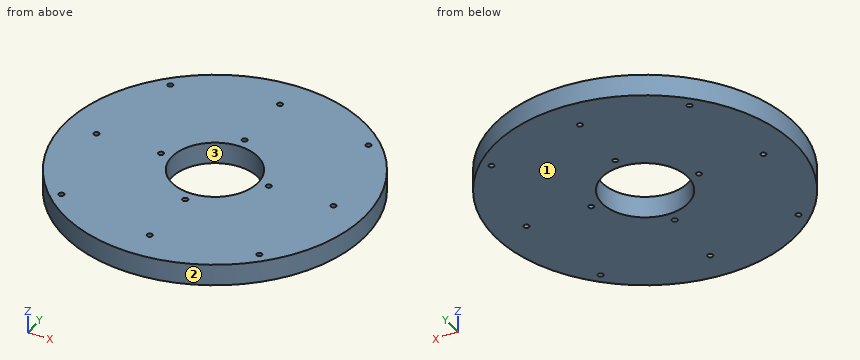
```python
from build123d import *

# Parameters (mm, degrees)
F0_R     = 140
F1_DEPTH = 20
F3_DEPTH = 20.001
F5_DEPTH = 25
F6_R     = 40
F7_DEPTH = 25
F9_DEPTH = 25


with BuildPart() as f1:
    # F0 (on Top) → F1 (new body)
    with BuildSketch(Plane.XY):
        Circle(F0_R)
    extrude(amount=F1_DEPTH)

    # F2 (on face) → F3 (cut, through all)
    with BuildSketch(Plane.XY.offset(20)):
        with BuildLine():
            ThreePointArc((-2.4998385795, 109.9715909091), (0, 110), (2.4998385795, 109.9715909091))
            ThreePointArc((2.4998385795, 109.9715909091), (2.4999596445, 109.9857952252), (2.5, 110))
            ThreePointArc((2.5, 110), (-0.0142047748, 112.4999596445), (-2.4998385795, 109.9715909091))
        make_face()
        with BuildLine():
            ThreePointArc((-2.4998385795, 109.9715909091), (0, 107.5), (2.4998385795, 109.9715909091))
            ThreePointArc((2.4998385795, 109.9715909091), (0, 110), (-2.4998385795, 109.9715909091))
        make_face()
        with BuildLine():
            ThreePointArc((109.9715909091, 2.4998385795), (109.992897498, 1.25), (110, 0))
            ThreePointArc((110, 0), (109.992897498, -1.25), (109.9715909091, -2.4998385795))
            ThreePointArc((109.9715909091, -2.4998385795), (111.7576941248, -1.7777827099), (112.5, 0))
            ThreePointArc((112.5, 0), (111.7576941248, 1.7777827099), (109.9715909091, 2.4998385795))
        make_face()
        with BuildLine():
            ThreePointArc((109.9715909091, -2.4998385795), (109.992897498, -1.25), (110, 0))
            ThreePointArc((110, 0), (109.992897498, 1.25), (109.9715909091, 2.4998385795))
            ThreePointArc((109.9715909091, 2.4998385795), (107.5, 0), (109.9715909091, -2.4998385795))
        make_face()
        with BuildLine():
            ThreePointArc((2.5, -110), (2.4999596445, -109.9857952252), (2.4998385795, -109.9715909091))
            ThreePointArc((2.4998385795, -109.9715909091), (0, -110), (-2.4998385795, -109.9715909091))
            ThreePointArc((-2.4998385795, -109.9715909091), (-0.0142047748, -112.4999596445), (2.5, -110))
        make_face()
        with BuildLine():
            ThreePointArc((-2.4998385795, -109.9715909091), (0, -110), (2.4998385795, -109.9715909091))
            ThreePointArc((2.4998385795, -109.9715909091), (0, -107.5), (-2.4998385795, -109.9715909091))
        make_face()
        with BuildLine():
            ThreePointArc((-107.5, 0), (-108.2222172901, 1.7576941248), (-109.9715909091, 2.4998385795))
            ThreePointArc((-109.9715909091, 2.4998385795), (-110, 0), (-109.9715909091, -2.4998385795))
            ThreePointArc((-109.9715909091, -2.4998385795), (-108.2222172901, -1.7576941248), (-107.5, 0))
        make_face()
        with BuildLine():
            ThreePointArc((-109.9715909091, -2.4998385795), (-110, 0), (-109.9715909091, 2.4998385795))
            ThreePointArc((-109.9715909091, 2.4998385795), (-112.5, 0), (-109.9715909091, -2.4998385795))
        make_face()
    extrude(amount=-F3_DEPTH, mode=Mode.SUBTRACT)

    # F4 (on face) → F5 (cut)
    with BuildSketch(Plane.XY.offset(20)):
        with BuildLine():
            ThreePointArc((-89.4238815543, 91.9238815543), (-89.6096098032, 92.8694746286), (-90.139198564, 93.6745690262))
            ThreePointArc((-90.139198564, 93.6745690262), (-91.0357485398, 92.8035154927), (-91.9238815543, 91.9238815543))
            Line((-91.9238815543, 91.9238815543), (-90.1561146013, 90.1561146013))
            ThreePointArc((-90.1561146013, 90.1561146013), (-89.614182723, 90.9671729733), (-89.4238815543, 91.9238815543))
        make_face()
        with BuildLine():
            ThreePointArc((-93.6745690262, 90.139198564), (-91.9118621846, 89.4239104475), (-90.1561146013, 90.1561146013))
            Line((-90.1561146013, 90.1561146013), (-91.9238815543, 91.9238815543))
            ThreePointArc((-91.9238815543, 91.9238815543), (-92.8035154927, 91.0357485398), (-93.6745690262, 90.139198564))
        make_face()
        with BuildLine():
            ThreePointArc((-91.9238815543, 91.9238815543), (-91.0357485398, 92.8035154927), (-90.139198564, 93.6745690262))
            ThreePointArc((-90.139198564, 93.6745690262), (-93.6916485072, 93.6916485072), (-93.6745690262, 90.139198564))
            ThreePointArc((-93.6745690262, 90.139198564), (-92.8035154927, 91.0357485398), (-91.9238815543, 91.9238815543))
        make_face()
        with BuildLine():
            ThreePointArc((91.9238815543, 91.9238815543), (92.8035154927, 91.0357485398), (93.6745690262, 90.139198564))
            ThreePointArc((93.6745690262, 90.139198564), (94.228954078, 90.9560795807), (94.4238815543, 91.9238815543))
            ThreePointArc((94.4238815543, 91.9238815543), (92.8694746286, 94.2381533053), (90.139198564, 93.6745690262))
            ThreePointArc((90.139198564, 93.6745690262), (91.0357485398, 92.8035154927), (91.9238815543, 91.9238815543))
        make_face()
        with BuildLine():
            ThreePointArc((90.1561146013, 90.1561146013), (91.9118621846, 89.4239104475), (93.6745690262, 90.139198564))
            ThreePointArc((93.6745690262, 90.139198564), (92.8035154927, 91.0357485398), (91.9238815543, 91.9238815543))
            Line((91.9238815543, 91.9238815543), (90.1561146013, 90.1561146013))
        make_face()
        with BuildLine():
            Line((90.1561146013, 90.1561146013), (91.9238815543, 91.9238815543))
            ThreePointArc((91.9238815543, 91.9238815543), (91.0357485398, 92.8035154927), (90.139198564, 93.6745690262))
            ThreePointArc((90.139198564, 93.6745690262), (89.4239104475, 91.9118621846), (90.1561146013, 90.1561146013))
        make_face()
        with BuildLine():
            ThreePointArc((94.4238815543, -91.9238815543), (94.228954078, -90.9560795807), (93.6745690262, -90.139198564))
            ThreePointArc((93.6745690262, -90.139198564), (92.8035154927, -91.0357485398), (91.9238815543, -91.9238815543))
            ThreePointArc((91.9238815543, -91.9238815543), (91.0357485398, -92.8035154927), (90.139198564, -93.6745690262))
            ThreePointArc((90.139198564, -93.6745690262), (92.8694746286, -94.2381533053), (94.4238815543, -91.9238815543))
        make_face()
        with BuildLine():
            ThreePointArc((91.9238815543, -91.9238815543), (92.8035154927, -91.0357485398), (93.6745690262, -90.139198564))
            ThreePointArc((93.6745690262, -90.139198564), (91.9118621846, -89.4239104475), (90.1561146013, -90.1561146013))
            Line((90.1561146013, -90.1561146013), (91.9238815543, -91.9238815543))
        make_face()
        with BuildLine():
            ThreePointArc((90.139198564, -93.6745690262), (91.0357485398, -92.8035154927), (91.9238815543, -91.9238815543))
            Line((91.9238815543, -91.9238815543), (90.1561146013, -90.1561146013))
            ThreePointArc((90.1561146013, -90.1561146013), (89.4239104475, -91.9118621846), (90.139198564, -93.6745690262))
        make_face()
        with BuildLine():
            ThreePointArc((-89.4238815543, -91.9238815543), (-89.614182723, -90.9671729733), (-90.1561146013, -90.1561146013))
            Line((-90.1561146013, -90.1561146013), (-91.9238815543, -91.9238815543))
            ThreePointArc((-91.9238815543, -91.9238815543), (-91.0357485398, -92.8035154927), (-90.139198564, -93.6745690262))
            ThreePointArc((-90.139198564, -93.6745690262), (-89.6096098032, -92.8694746286), (-89.4238815543, -91.9238815543))
        make_face()
        with BuildLine():
            ThreePointArc((-93.6745690262, -90.139198564), (-93.6916485072, -93.6916485072), (-90.139198564, -93.6745690262))
            ThreePointArc((-90.139198564, -93.6745690262), (-91.0357485398, -92.8035154927), (-91.9238815543, -91.9238815543))
            ThreePointArc((-91.9238815543, -91.9238815543), (-92.8035154927, -91.0357485398), (-93.6745690262, -90.139198564))
        make_face()
        with BuildLine():
            Line((-91.9238815543, -91.9238815543), (-90.1561146013, -90.1561146013))
            ThreePointArc((-90.1561146013, -90.1561146013), (-91.9118621846, -89.4239104475), (-93.6745690262, -90.139198564))
            ThreePointArc((-93.6745690262, -90.139198564), (-92.8035154927, -91.0357485398), (-91.9238815543, -91.9238815543))
        make_face()
    extrude(amount=-F5_DEPTH, mode=Mode.SUBTRACT)

    # F6 (on face) → F7 (cut)
    with BuildSketch(Plane.XY.offset(20)):
        Circle(F6_R)
    extrude(amount=-F7_DEPTH, mode=Mode.SUBTRACT)

    # F8 (on face) → F9 (cut)
    with BuildSketch(Plane.XY.offset(20)):
        with BuildLine():
            ThreePointArc((-2.4992186279, 49.9375), (0, 50), (2.4992186279, 49.9375))
            ThreePointArc((2.4992186279, 49.9375), (2.4998046493, 49.9687475579), (2.5, 50))
            ThreePointArc((2.5, 50), (-0.0312524421, 52.4998046493), (-2.4992186279, 49.9375))
        make_face()
        with BuildLine():
            ThreePointArc((-2.4992186279, 49.9375), (0, 47.5), (2.4992186279, 49.9375))
            ThreePointArc((2.4992186279, 49.9375), (0, 50), (-2.4992186279, 49.9375))
        make_face()
        with BuildLine():
            ThreePointArc((-47.5, 0), (-48.2102723671, 1.7455300055), (-49.9375, 2.4992186279))
            ThreePointArc((-49.9375, 2.4992186279), (-50, 0), (-49.9375, -2.4992186279))
            ThreePointArc((-49.9375, -2.4992186279), (-48.2102723671, -1.7455300055), (-47.5, 0))
        make_face()
        with BuildLine():
            ThreePointArc((-49.9375, -2.4992186279), (-50, 0), (-49.9375, 2.4992186279))
            ThreePointArc((-49.9375, 2.4992186279), (-52.5, 0), (-49.9375, -2.4992186279))
        make_face()
        with BuildLine():
            ThreePointArc((2.5, -50), (2.4998046493, -49.9687475579), (2.4992186279, -49.9375))
            ThreePointArc((2.4992186279, -49.9375), (0, -50), (-2.4992186279, -49.9375))
            ThreePointArc((-2.4992186279, -49.9375), (-0.0312524421, -52.4998046493), (2.5, -50))
        make_face()
        with BuildLine():
            ThreePointArc((-2.4992186279, -49.9375), (0, -50), (2.4992186279, -49.9375))
            ThreePointArc((2.4992186279, -49.9375), (0, -47.5), (-2.4992186279, -49.9375))
        make_face()
        with BuildLine():
            ThreePointArc((49.9375, 2.4992186279), (49.9843725578, 1.25), (50, 0))
            ThreePointArc((50, 0), (49.9843725578, -1.25), (49.9375, -2.4992186279))
            ThreePointArc((49.9375, -2.4992186279), (51.7455300055, -1.7897276329), (52.5, 0))
            ThreePointArc((52.5, 0), (51.7455300055, 1.7897276329), (49.9375, 2.4992186279))
        make_face()
        with BuildLine():
            ThreePointArc((49.9375, -2.4992186279), (49.9843725578, -1.25), (50, 0))
            ThreePointArc((50, 0), (49.9843725578, 1.25), (49.9375, 2.4992186279))
            ThreePointArc((49.9375, 2.4992186279), (47.5, 0), (49.9375, -2.4992186279))
        make_face()
    extrude(amount=-F9_DEPTH, mode=Mode.SUBTRACT)


solid = f1.part
```
Check sheet for the modelled part. Datum: model origin and axes. Units: mm. Face numbers are marked on the shaded views. Coordinates: 2 decimals unless noted, no trailing zeros. Order: outer loops, then holes, each group sorted by start corner. A loop starts at its lowest first (then second) coordinate and runs counter-clockwise, first axis right, second up. Notation, with made-up numbers: M 22.25,49 L 30.25,49 A32 ccw 30.25,78 Z; hole C 72,74 d7. An arc over 180 degrees is marked long. Write each question's results on one line, items separated by ' | '. Start each with the question number.
1. Cross-section at D-D on x = -69. Record the cut outline in (y, z), and give its area (3 significant figures).
2. Cross-section at C-C on y = -70. Record the cut outline in (x, z), and give its area (3 significant figures).
3. Go/stop test with flat-tipped pins: P1, Ø4, axis at x = -102.5, z = 6, coming from the +Y side; P2, Ø6, axis at x = -32, z = 11, coming from the +Y side; P3, Ø5, axis at x = 4.5, z = 17.5, coming from the -Y side. Record where each tip stops, or that it passes through.
4. Cross-section at A-A on x = -16.5. Record the cut outline in (y, z).
5. Cross-section at B-B on y = 7. Record the cut outline in (x, z).
6. Mould release check, pull along X, two halves, no side actions. Record for the marked faces 1, 2 and 3: +X half, -X half, draft (parallel to the pull), parting line (faces both ways), or undercut.
7. Material ranges on probe 1 along X at (y, z) = (50.5, 10.75); probe 2 along Y at (x, z) = (-10.5, 3.75); probe 3 along X at (y, z) = (6.5, 17.75), recorded low to high.
Checks:
1) outline: M -121.82,0 L 121.82,0 L 121.82,20 L -121.82,20 Z | area: 4,870 mm²
2) outline: M -121.24,0 L 121.24,0 L 121.24,20 L -121.24,20 Z | area: 4,850 mm²
3) P1: stops at y = 97.47 | P2: stops at y = 136.96 | P3: stops at y = -139.99
4) outline: M -139.02,0 L -36.44,0 L -36.44,20 L -139.02,20 Z; M 36.44,0 L 139.02,0 L 139.02,20 L 36.44,20 Z
5) outline: M -139.82,0 L -39.38,0 L -39.38,20 L -139.82,20 Z; M 39.38,0 L 139.82,0 L 139.82,20 L 39.38,20 Z
6) face 1: draft | face 2: parting line | face 3: undercut
7) probe 1: x = -130.57 to -2.45, 2.45 to 130.57 | probe 2: y = -139.61 to -38.6, 38.6 to 139.61 | probe 3: x = -139.85 to -39.47, 39.47 to 139.85
